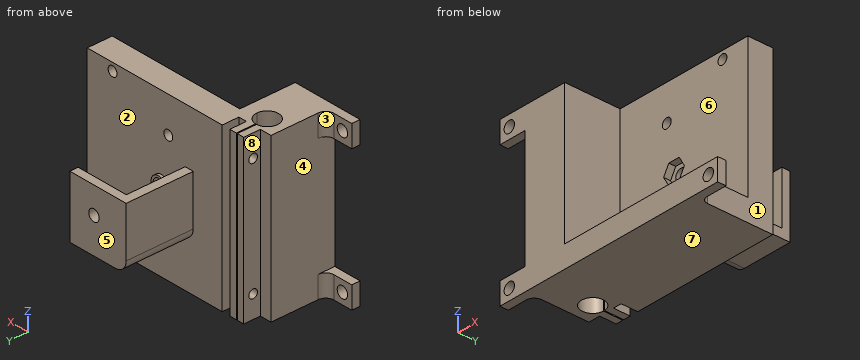
```python
from build123d import *

# Parameters (mm, degrees)
SKETCH1_W           = 66
SKETCH1_H           = 58.3
SKETCH1_R           = 2.05
BOSS_EXTRUDE1_DEPTH = 29
CUT_EXTRUDE1_START  = -29
CUT_EXTRUDE1_DEPTH  = 20
SKETCH6_W           = 10
SKETCH6_H           = 7.9
SKETCH6_R           = 2.05
BOSS_EXTRUDE2_DEPTH = 3
BOSS_EXTRUDE4_DEPTH = 7.9
BOSS_EXTRUDE5_START = -50.4
BOSS_EXTRUDE5_DEPTH = 7.9
CUT_EXTRUDE4_START  = -58.3
SKETCH8_R           = 4.05
CUT_EXTRUDE4_DEPTH  = 58.3
CUT_EXTRUDE5_REACH  = 80.031
SKETCH10_W          = 3
SKETCH10_H          = 6
SKETCH10_W_2        = 4.2
SKETCH10_W_3        = 0.4
SKETCH10_H_2        = 7.617508416
CUT_EXTRUDE6_REACH  = 84.74
SKETCH11_R          = 1.55
CUT_EXTRUDE7_DEPTH  = 2.5
BOSS_EXTRUDE6_DEPTH = 21.2
SKETCH14_R          = 2.05
BOSS_EXTRUDE7_DEPTH = 3
BOSS_EXTRUDE8_START = -4
SKETCH15_R          = 2.85
SKETCH15_R_2        = 2.05
BOSS_EXTRUDE8_DEPTH = 1
BOSS_EXTRUDE9_START = -24.2
SKETCH15_2_R        = 2.85
SKETCH15_2_R_2      = 2.05
BOSS_EXTRUDE9_DEPTH = 1
SKETCH16_W          = 60.451877866
SKETCH16_H          = 7.9
CUT_EXTRUDE8_DEPTH  = 20
SKETCH19_R          = 1.75
CUT_EXTRUDE9_DEPTH  = 9


with BuildPart() as part:
    # Sketch1 → Boss-Extrude1 (new body)
    with BuildSketch(Plane(origin=(0, 0, 0), x_dir=(1, 0, 0), z_dir=(0, 1, 0))):
        Rectangle(SKETCH1_W, SKETCH1_H)
        with Locations(Location((-3.85, 0, 0), (0, 0, 90))):
            Circle(SKETCH1_R, mode=Mode.SUBTRACT)
    extrude(amount=BOSS_EXTRUDE1_DEPTH)

    # Sketch3 → Cut-Extrude1 (cut)
    with BuildSketch(Plane(origin=(0, 29, 0), x_dir=(1, 0, 0), z_dir=(0, 1, 0)).offset(CUT_EXTRUDE1_START)):
        Polygon((-33, 21.25), (-33, -21.25), (17.4, -21.25), (17.4, 21.25), (-25.1, 21.25), align=None)
    extrude(amount=CUT_EXTRUDE1_DEPTH, mode=Mode.SUBTRACT)

    # Sketch6 → Boss-Extrude2 (add)
    # profile 1 of 4: a face of its own
    with BuildSketch(Plane.XZ):
        with Locations((-38, 25.2)):
            Rectangle(SKETCH6_W, SKETCH6_H)
        with Locations(Location((-39.3, 25.2, 0), (0, 0, 270))):
            Circle(SKETCH6_R, mode=Mode.SUBTRACT)
    # profile 2 of 4: a face of its own
    with BuildSketch(Plane.XZ):
        with Locations((-38, -25.2)):
            Rectangle(SKETCH6_W, SKETCH6_H)
        with Locations(Location((-39.3, -25.2, 0), (0, 0, 270))):
            Circle(SKETCH6_R, mode=Mode.SUBTRACT)
    # profile 3 of 4: a face of its own
    with BuildSketch(Plane.XZ):
        with Locations((38, 25.2)):
            Rectangle(SKETCH6_W, SKETCH6_H)
        with Locations(Location((39.3, 25.2, 0), (0, 0, 270))):
            Circle(SKETCH6_R, mode=Mode.SUBTRACT)
    # profile 4 of 4: a face of its own
    with BuildSketch(Plane.XZ):
        with Locations((38, -25.2)):
            Rectangle(SKETCH6_W, SKETCH6_H)
        with Locations(Location((39.3, -25.2, 0), (0, 0, 270))):
            Circle(SKETCH6_R, mode=Mode.SUBTRACT)
    extrude(amount=-BOSS_EXTRUDE2_DEPTH)

    # Sketch7 → Boss-Extrude4 (add)
    with BuildSketch(Plane(origin=(0, 0, -29.15), x_dir=(-1, 0, 0), z_dir=(0, 0, -1))):
        with BuildLine():
            ThreePointArc((35.5, 3), (33.732233047, 3.732233047), (33, 5.5))
            Line((33, 5.5), (33, 3))
            Line((33, 3), (35.5, 3))
        make_face()
        with BuildLine():
            ThreePointArc((-33, 6), (-33.878679656, 3.878679656), (-36, 3))
            Line((-36, 3), (-33, 3))
            Line((-33, 3), (-33, 6))
        make_face()
    extrude(amount=-BOSS_EXTRUDE4_DEPTH)

    # Sketch7<5> → Boss-Extrude5 (add)
    with BuildSketch(Plane(origin=(0, 0, -29.15), x_dir=(-1, 0, 0), z_dir=(0, 0, -1)).offset(BOSS_EXTRUDE5_START)):
        with BuildLine():
            ThreePointArc((35.5, 3), (33.732233047, 3.732233047), (33, 5.5))
            Line((33, 5.5), (33, 3))
            Line((33, 3), (35.5, 3))
        make_face()
        with BuildLine():
            ThreePointArc((-33, 6), (-33.878679656, 3.878679656), (-36, 3))
            Line((-36, 3), (-33, 3))
            Line((-33, 3), (-33, 6))
        make_face()
    extrude(amount=-BOSS_EXTRUDE5_DEPTH)

    # Sketch8 → Cut-Extrude4 (cut)
    with BuildSketch(Plane.XY.offset(29.15).offset(CUT_EXTRUDE4_START)):
        with Locations(Location((26.05, 18, 0), (0, 0, 180))):
            Circle(SKETCH8_R)
    extrude(amount=CUT_EXTRUDE4_DEPTH, mode=Mode.SUBTRACT)

    # Sketch10 → Cut-Extrude5 (cut, up to next)
    with BuildSketch(Plane(origin=(0, 0, -29.15), x_dir=(-1, 0, 0), z_dir=(0, 0, -1)), mode=Mode.PRIVATE) as cut_extrude5_sk1:
        with Locations((-21.8, 26)):
            Rectangle(SKETCH10_W, SKETCH10_H)
    cut_extrude5_tool1 = extrude(cut_extrude5_sk1.sketch, amount=-CUT_EXTRUDE5_REACH, mode=Mode.PRIVATE) & part.part
    # Sketch10 → Cut-Extrude5 (cut, up to next)
    with BuildSketch(Plane(origin=(0, 0, -29.15), x_dir=(-1, 0, 0), z_dir=(0, 0, -1)), mode=Mode.PRIVATE) as cut_extrude5_sk2:
        with Locations((-30.9, 26)):
            Rectangle(SKETCH10_W_2, SKETCH10_H)
    cut_extrude5_tool2 = extrude(cut_extrude5_sk2.sketch, amount=-CUT_EXTRUDE5_REACH, mode=Mode.PRIVATE) & part.part
    # Sketch10 → Cut-Extrude5 (cut, up to next)
    with BuildSketch(Plane(origin=(0, 0, -29.15), x_dir=(-1, 0, 0), z_dir=(0, 0, -1)), mode=Mode.PRIVATE) as cut_extrude5_sk3:
        with Locations((-26.05, 25.191245792)):
            Rectangle(SKETCH10_W_3, SKETCH10_H_2)
    cut_extrude5_tool3 = extrude(cut_extrude5_sk3.sketch, amount=-CUT_EXTRUDE5_REACH, mode=Mode.PRIVATE) & part.part
    add(cut_extrude5_tool1.solids().sort_by_distance((21.8, 26, -29.15))[0], mode=Mode.SUBTRACT)
    add(cut_extrude5_tool2.solids().sort_by_distance((30.9, 26, -29.15))[0], mode=Mode.SUBTRACT)
    add(cut_extrude5_tool3.solids().sort_by_distance((26.05, 25.191246, -29.15))[0], mode=Mode.SUBTRACT)

    # Cut-Extrude6: up to this face of the body (flat: up to its plane)
    cut_extrude6_end = Plane(part.part.faces().sort_by_distance((23.3, 26, 0))[0])
    # Sketch11 → Cut-Extrude6 (cut, up to the picked face)
    with BuildSketch(Plane(origin=(28.8, 0, 0), x_dir=(0, 0, -1), z_dir=(1, 0, 0)), mode=Mode.PRIVATE) as cut_extrude6_sk1:
        with Locations((-21.15, 25.6)):
            Circle(SKETCH11_R)
    cut_extrude6_tool1 = split(extrude(cut_extrude6_sk1.sketch, amount=-CUT_EXTRUDE6_REACH, mode=Mode.PRIVATE), bisect_by=cut_extrude6_end, keep=Keep.BOTH, mode=Mode.PRIVATE)
    # Sketch11 → Cut-Extrude6 (cut, up to the picked face)
    with BuildSketch(Plane(origin=(28.8, 0, 0), x_dir=(0, 0, -1), z_dir=(1, 0, 0)), mode=Mode.PRIVATE) as cut_extrude6_sk2:
        with Locations((21.15, 25.6)):
            Circle(SKETCH11_R)
    cut_extrude6_tool2 = split(extrude(cut_extrude6_sk2.sketch, amount=-CUT_EXTRUDE6_REACH, mode=Mode.PRIVATE), bisect_by=cut_extrude6_end, keep=Keep.BOTH, mode=Mode.PRIVATE)
    add(cut_extrude6_tool1.solids().sort_by(Axis((28.8, 25.6, 21.15), (-1, 0, 0)))[0], mode=Mode.SUBTRACT)
    add(cut_extrude6_tool2.solids().sort_by(Axis((28.8, 25.6, -21.15), (-1, 0, 0)))[0], mode=Mode.SUBTRACT)

    # Sketch12 → Cut-Extrude7 (cut)
    with BuildSketch(Plane.XZ.offset(-20)):
        Polygon((-7.95, 0), (-5.9, -3.550704156), (-1.8, -3.550704156), (0.25, 0), (-1.8, 3.550704156), (-5.9, 3.550704156), align=None)
    extrude(amount=-CUT_EXTRUDE7_DEPTH, mode=Mode.SUBTRACT)

    # Sketch13 → Boss-Extrude6 (add)
    with BuildSketch(Plane(origin=(0, 29, 0), x_dir=(1, 0, 0), z_dir=(0, 1, 0))):
        with BuildLine():
            Line((-13.35, 9.5), (-13.35, 12.7))
            Line((-13.35, 12.7), (4.65, 12.7))
            ThreePointArc((4.65, 12.7), (7.619848481, 11.469848481), (8.85, 8.5))
            Line((8.85, 8.5), (8.85, -9.5))
            Line((8.85, -9.5), (5.65, -9.5))
            Line((5.65, -9.5), (5.65, 6.3))
            ThreePointArc((5.65, 6.3), (4.7127417, 8.5627417), (2.45, 9.5))
            Line((2.45, 9.5), (-13.35, 9.5))
        make_face()
    extrude(amount=BOSS_EXTRUDE6_DEPTH)

    # Sketch14 → Boss-Extrude7 (add)
    with BuildSketch(Plane(origin=(0, 50.2, 0), x_dir=(1, 0, 0), z_dir=(0, 1, 0))):
        with BuildLine():
            Line((-13.35, 12.7), (4.65, 12.7))
            ThreePointArc((4.65, 12.7), (7.619848481, 11.469848481), (8.85, 8.5))
            Line((8.85, 8.5), (8.85, -9.5))
            Line((8.85, -9.5), (-13.35, -9.5))
            Line((-13.35, -9.5), (-13.35, 12.7))
        make_face()
        with Locations(Location((-3.85, 0, 0), (0, 0, 90))):
            Circle(SKETCH14_R, mode=Mode.SUBTRACT)
    extrude(amount=BOSS_EXTRUDE7_DEPTH)

    # Sketch15 → Boss-Extrude8 (add)
    with BuildSketch(Plane(origin=(0, 53.2, 0), x_dir=(1, 0, 0), z_dir=(0, 1, 0)).offset(BOSS_EXTRUDE8_START)):
        with Locations(Location((-3.85, 0, 0), (0, 0, 270))):
            Circle(SKETCH15_R)
        with Locations(Location((-3.85, 0, 0), (0, 0, 90))):
            Circle(SKETCH15_R_2, mode=Mode.SUBTRACT)
    extrude(amount=BOSS_EXTRUDE8_DEPTH)

    # Sketch15<2> → Boss-Extrude9 (add)
    with BuildSketch(Plane(origin=(0, 53.2, 0), x_dir=(1, 0, 0), z_dir=(0, 1, 0)).offset(BOSS_EXTRUDE9_START)):
        with Locations(Location((-3.85, 0, 0), (0, 0, 270))):
            Circle(SKETCH15_2_R)
        with Locations(Location((-3.85, 0, 0), (0, 0, 90))):
            Circle(SKETCH15_2_R_2, mode=Mode.SUBTRACT)
    extrude(amount=BOSS_EXTRUDE9_DEPTH)


with BuildPart() as body_2:
    # Mirror2: mirrored copy
    add(part.part.mirror(Plane(origin=(-43, 3, -21.25), x_dir=(0, 0, 1), z_dir=(-1, 0, 0))))

    # Sketch16 → Cut-Extrude8 (cut)
    with BuildSketch(Plane.XZ):
        with Locations((-73.174061067, 25.2)):
            Rectangle(SKETCH16_W, SKETCH16_H)
    extrude(amount=-CUT_EXTRUDE8_DEPTH, mode=Mode.SUBTRACT)

    # Sketch19 → Cut-Extrude9 (cut)
    with BuildSketch(Plane.XZ.offset(-20)):
        with Locations(Location((-85, 16.35, 0), (0, 0, 270))):
            Circle(SKETCH19_R)
        with Locations(Location((-63, 26.35, 0), (0, 0, 270))):
            Circle(SKETCH19_R)
    extrude(amount=-CUT_EXTRUDE9_DEPTH, mode=Mode.SUBTRACT)


solid = body_2.part
```
Part model, mm, in its own coordinate system. Face numbers are marked on the shaded views. A direction names the side the tool comes from. Round coordinates to 2 decimals unless told otherwise and drop trailing zeros. Write each loop counter-clockwise with the first axis right and the second up, starting at its lowest first coordinate (ties: lowest second). Pieces come first, ordered by that corner, then holes. Notation, with made-up numbers: (-40, 14.5) -> (2, 14.5) arc R36 ccw to (2, 52.5) -> close; hole circle Ø3 at (84, 72). An arc over 180 degrees is marked (long way). Return JSON: item names as keys, results as strings. Group by question number.
Q1. Saw through at C-C on x = -63. Write the cut outline in (y, z).
Q2. Saw through at B-B on y = 42. Write the cut outline in (x, z), plus the area to 3 significant figures.
Q3. Probe L1, parallel to X at y = 1.85, z = -25.2; L2, parallel to X at y = 28, z = 20.5; L3, parallel to Z at x = -82, y = 27. List the from-to ranges inside material, lowest first. Write a range as [from, to].
Q4. Pin check, flat tips, straight feed: pin 1 (2 mm diameter, centred on x = -115.5, z = -22, fed in from +Y); pin 2 (3 mm diameter, centred on y = 25.5, z = 8.5, fed in from -X); pin 3 (2 mm diameter, centred on x = -126, z = -24, fed in from +Y); pin 4 (3 mm diameter, centred on x = -63, z = 26.35, fed in from -Y). Stop position of each tip, or through.
Q5. Mould opens along Y. For the marked faces 1, 2 and 3 say: pulls with the +Y half, pulls with the -Y half, needs draft (parallel to the pull), parting line crosses it, or undercut.
Q6. Which spindle directions (+Z, -Z, +X, -X, +Y, -Y) get a long thin tool onto all of the face, cutting with end or side? Do the marked faces 4, 5, 6, 7 and 8. Say none if no direction does.
Q7. Saw through at D-D on x = -82.15. State how many separate pieces and enclosed holes the cut face has, plus the area to 3 significant figures.
Q8. Saw through at A-A on x = -125.3. Write the cut outline in (y, z), plus the area to 3 significant figures.
Answer:
{
 "1": {"outline": "(0, -29.15) -> (29, -29.15) -> (29, 24.6) -> (20, 24.6) -> (20, -21.25) -> (0, -21.25) -> close; (20, 28.1) -> (29, 28.1) -> (29, 29.15) -> (20, 29.15) -> close"},
 "2": {"outline": "(-94.85, -8.5) arc R4.2 ccw to (-90.65, -12.7) -> (-72.65, -12.7) -> (-72.65, -9.5) -> (-88.45, -9.5) arc R3.2 cw to (-91.65, -6.3) -> (-91.65, 9.5) -> (-94.85, 9.5) -> close", "area": "130 mm2"},
 "3": {"L1": "[-129, -127.35], [-123.25, -48.75], [-44.65, -43]", "L2": "[-114.8, -112.25], [-111.85, -109.3], [-106.3, -53]", "L3": "[-29.15, -2.04], [2.04, 29.15]"},
 "4": {"pin 1": "y = 29", "pin 2": "x = -114.8", "pin 3": "y = 3", "pin 4": "through"},
 "5": {"face 1": "needs draft", "face 2": "undercut", "face 3": "pulls with the +Y half"},
 "6": {"face 4": "-X, +Y", "face 5": "+Z, -Z, +X, -X, +Y", "face 6": "+Z, +X, -Y", "face 7": "-Z, +X, -X, +Y, -Y", "face 8": "+Z, -Z, -X, +Y"},
 "7": {"separate pieces": "3", "enclosed holes": "0", "area": "764 mm2"},
 "8": {"outline": "(0, -29.15) -> (3, -29.15) -> (3, -27.25) -> (0, -27.25) -> close; (0, -23.15) -> (3, -23.15) -> (3, -21.25) -> (0, -21.25) -> close; (0, 21.25) -> (3, 21.25) -> (3, 23.15) -> (0, 23.15) -> close; (0, 27.25) -> (3, 27.25) -> (3, 29.15) -> (0, 29.15) -> close", "area": "22.8 mm2"}
}
